The listing builds one solid part. Answer for the finished solid, in the listing's coordinates (mm). Coordinates: 2 decimals unless noted, no trailing zeros. Order: outer loops, then holes, each group sorted by start corner. A loop starts at its lowest first (then second) coordinate and runs counter-clockwise, first axis right, second up. Notation, with made-up numbers: (56.5, 60.25) -> (89.5, 60.25) arc R23 cw to (89.5, 99.25) -> close; hole circle Ø7 at (51.25, -9). An arc over 180 degrees is marked (long way). Answer in a Markdown table with one row per item.
```python
from build123d import *

# Parameters (mm, degrees)
F1_DEPTH = 5
F2_R     = 4
F3_DEPTH = 5


with BuildPart() as f1:
    # F0 (on Front) → F1 (new body)
    with BuildSketch(Plane.XZ):
        with BuildLine():
            Line((15, 7.5), (-15, 7.5))
            ThreePointArc((-15, 7.5), (-22.5, 0), (-15, -7.5))
            Line((-15, -7.5), (15, -7.5))
            ThreePointArc((15, -7.5), (22.5, 0), (15, 7.5))
        make_face()
    extrude(amount=F1_DEPTH)

    # F2 (on face) → F3 (cut)
    with BuildSketch(Plane.XZ.offset(5)):
        with Locations((-15, 0)):
            Circle(F2_R)
        with Locations((15, 0)):
            Circle(F2_R)
    extrude(amount=-F3_DEPTH, mode=Mode.SUBTRACT)


solid = f1.part
```
(1) A cutting plane is placed at C-C, the plane y = -3.1. Determine the outline of the cut face in (x, z).
Check values:
| item | result |
|---|---|
| outline | (-15, -7.5) -> (15, -7.5) arc R7.5 ccw to (15, 7.5) -> (-15, 7.5) arc R7.5 ccw to start; hole circle Ø8 at (-15, 0); hole circle Ø8 at (15, 0) |
(2) A cutting plane is placed at B-B, the plane x = 18. Determine the outline of the cut face in (y, z).
Check values:
| item | result |
|---|---|
| outline | (-5, -6.87) -> (0, -6.87) -> (0, -2.65) -> (-5, -2.65) -> close; (-5, 2.65) -> (0, 2.65) -> (0, 6.87) -> (-5, 6.87) -> close |
(3) A cutting plane is placed at D-D, the plane z = 5.25. Determine the outline of the cut face in (x, y), then the cut area to 3 significant figures.
Check values:
| item | result |
|---|---|
| outline | (-20.36, -5) -> (20.36, -5) -> (20.36, 0) -> (-20.36, 0) -> close |
| area | 204 mm² |
(4) For a pull along X with two mould halves and no side action, classify faces 1 (the flat face through (0, -5, 0)), 2 (the cylindrical face through (22.5, -2.46, -0.16)), 3 (the cylindrical face through (-19, -3, 0)), 4 (the cylindrical face through (11, -3, 0)) as released by +X, released by -X, zero draft, split by the parting line, or undercut.
Check values:
| item | result |
|---|---|
| face 1 | zero draft |
| face 2 | released by +X |
| face 3 | undercut |
| face 4 | undercut |
(5) A flat-ended cylindrical pin translates along its axis: pin 1 (3 mm diameter, centred on x = -17.5, y = -2.5, fed in from -Z). Find the tip coordinate at first contact, or state that the pin passes through.
Check values:
| item | result |
|---|---|
| pin 1 | z = -7.43 |
(6) Find the intervals of material crossed by line 1 along Z through (x, y) = (-15, -1.7); line 2 along X through (y, z) = (-2.1, 1); line 3 along X through (y, z) = (-4.6, -2.5), in increasing order. Write a range as from..to.
Check values:
| item | result |
|---|---|
| line 1 | -7.5..-4, 4..7.5 |
| line 2 | -22.43..-18.87, -11.13..11.13, 18.87..22.43 |
| line 3 | -22.07..-18.12, -11.88..11.88, 18.12..22.07 |
(7) A cutting plane is placed at A-A, the plane z = 0. Determine the outline of the cut face in (x, y).
Check values:
| item | result |
|---|---|
| outline | (-22.5, -5) -> (-19, -5) -> (-19, 0) -> (-22.5, 0) -> close; (-11, -5) -> (11, -5) -> (11, 0) -> (-11, 0) -> close; (19, -5) -> (22.5, -5) -> (22.5, 0) -> (19, 0) -> close |
